Build history of the part. All positions in model axes, mm. Coordinates: 2 decimals unless noted, no trailing zeros. Order: outer loops, then holes, each group sorted by start corner. A loop starts at its lowest first (then second) coordinate and runs counter-clockwise, first axis right, second up. Notation, with made-up numbers: (11.25, 44.5) -> (60.25, 44.5) arc R24 cw to (60.25, 77.5) -> close; hole circle Ø1 at (89, -40). An arc over 180 degrees is marked (long way). Write each question's results on one line, items separated by ' | '.
from build123d import *

# Parameters (mm, degrees)
SKETCH1_W           = 51.054
SKETCH1_H           = 50.038
BOSS_EXTRUDE1_DEPTH = 17.272
CHAMFER1_SIZE       = 5
FILLET1_R           = 2.54
SKETCH2_R           = 2.159
CUT_EXTRUDE1_DEPTH  = 48.875253562


with BuildPart() as part:
    # Sketch1 → Boss-Extrude1 (new body)
    with BuildSketch(Plane(origin=(0, 0, 0), x_dir=(1, 0, 0), z_dir=(0, 1, 0))):
        with Locations((-10.305704367, -1.621856169)):
            Rectangle(SKETCH1_W, SKETCH1_H)
    extrude(amount=BOSS_EXTRUDE1_DEPTH)

    # Chamfer1
    chamfer1_edges = [part.edges().sort_by_distance(p)[0] for p in [
        (15.221295633, 8.636, -23.397143831),
        (15.221295633, 8.636, 26.640856169),
    ]]
    chamfer(chamfer1_edges, length=CHAMFER1_SIZE)

    # Fillet1
    fillet1_edges = [part.edges().sort_by_distance(p)[0] for p in [
        (-35.832704367, 8.636, -23.397143831),
        (-35.832704367, 8.636, 26.640856169),
    ]]
    fillet(fillet1_edges, radius=FILLET1_R)

    # Sketch2 → Cut-Extrude1 (cut, through all)
    with BuildSketch(Plane(origin=(0, 17.272, 0), x_dir=(1, 0, 0), z_dir=(0, 1, 0))):
        with Locations(Location((-25.672704367, 13.491143831, 0), (0, 0, 270))):
            Circle(SKETCH2_R)
        with Locations(Location((4.045295633, 13.491143831, 0), (0, 0, 270))):
            Circle(SKETCH2_R)
        with Locations(Location((4.045295633, -16.734856169, 0), (0, 0, 270))):
            Circle(SKETCH2_R)
        with Locations(Location((-25.672704367, -16.734856169, 0), (0, 0, 270))):
            Circle(SKETCH2_R)
    extrude(amount=-CUT_EXTRUDE1_DEPTH, mode=Mode.SUBTRACT)


solid = part.part
Item 1: Pull direction Z, two halves, no side cores. Call faces 1 (the flat face through (15.221, 9, 2)), 2 (the cylindrical face through (-23.852, 8.757, -12.33)), 3 (the cylindrical face through (-35.069, 8.757, 25.917)): released by +Z, released by -Z, zero draft, split by the parting line, or undercut.
Answer:
face 1: zero draft | face 2: undercut | face 3: released by +Z
Item 2: Slice it at C-C, the plane z = -20. List the corners of the cut face in (x, y), and give its area (3 significant figures).
Answer:
outline: (-35.83, 0) -> (13.62, 0) -> (13.62, 17.27) -> (-35.83, 17.27) -> close | area: 854 mm^2
Item 3: Drill centre lines: line 1 (Z direction, x = -25.5, y = 14.5); line 2 (X direction, y = 12.75, z = 16); line 3 (X direction, y = 15.75, z = 15.5). Where is each one in solid material? Low to high. Write a range as from..to.
Answer:
line 1: z = -23.4..-15.64, -11.34..14.58, 18.89..26.64 | line 2: x = -35.83..-27.7, -23.64..2.02, 6.08..15.22 | line 3: x = -35.83..-27.44, -23.9..2.27, 5.82..15.22
Item 4: Slice it at A-A, the plane z = -14. List the corners of the cut face in (x, y).
Answer:
outline: (-35.83, 0) -> (-27.77, 0) -> (-27.77, 17.27) -> (-35.83, 17.27) -> close; (-23.57, 0) -> (1.95, 0) -> (1.95, 17.27) -> (-23.57, 17.27) -> close; (6.14, 0) -> (15.22, 0) -> (15.22, 17.27) -> (6.14, 17.27) -> close
Item 5: Slice it at B-B, the plane y = 9.5. List the corners of the cut face in (x, z), and give its area (3 significant figures).
Answer:
outline: (-35.83, -20.86) arc R2.54 ccw to (-33.29, -23.4) -> (10.22, -23.4) -> (15.22, -18.4) -> (15.22, 21.64) -> (10.22, 26.64) -> (-33.29, 26.64) arc R2.54 ccw to (-35.83, 24.1) -> close; hole circle Ø4.32 at (-25.67, -13.49); hole circle Ø4.32 at (-25.67, 16.73); hole circle Ø4.32 at (4.05, -13.49); hole circle Ø4.32 at (4.05, 16.73) | area: 2,470 mm^2
Item 6: Pin check, flat tip, straight feed: pin 1 (4 mm diameter, centred on y = 15, z = -18.5, fed in from +X). Stop position of the tip, or through.
Answer:
pin 1: stops at x = 15.22
